Autodesk Inventor part; units mm, degrees
ref_plane "Start plane" through (0, 0, 0) normal (0, 0, 1) x (1, 0, 0)
ref_plane "End plane" through (0, 0, 300) normal (0, 0, 1) x (1, 0, 0)
ref_plane "Work Plane4" through (10, 0, 0) normal (-0.7071, 0, -0.7071) x (-0.7071, 0, 0.7071)
ref_plane "Start plane" through (0, 0, 0) normal (0, 0, 1) x (1, 0, 0)
ref_plane "End plane" through (0, 0, 300) normal (0, 0, 1) x (1, 0, 0)
sketch "Sketch" plane through (0, 0, 0) normal (0, 0, 1) x (1, 0, 0)
  line L0 (-10, -6) -> (-10, 6)
  line L1 (-6, 10) -> (6, 10)
  line L2 (10, 6) -> (10, -6)
  line L3 (6, -10) -> (-6, -10)
  arc A0 (-10, -6) -> (-6, -10) centre (-6, -6) ccw
  arc A1 (10, 6) -> (6, 10) centre (6, 6) ccw
  arc A2 (-6, 10) -> (-10, 6) centre (-6, 6) ccw
  arc A3 (6, -10) -> (10, -6) centre (6, -6) ccw
  arc A4 (-6, 8) -> (-8, 6) centre (-6, 6) ccw
  line L4 (-6, 8) -> (6, 8)
  arc A5 (8, 6) -> (6, 8) centre (6, 6) ccw
  line L5 (8, 6) -> (8, -6)
  arc A6 (6, -8) -> (8, -6) centre (6, -6) ccw
  line L6 (6, -8) -> (-6, -8)
  arc A7 (-8, -6) -> (-6, -8) centre (-6, -6) ccw
  line L7 (-8, -6) -> (-8, 6)
  line L8 (0, 15.1598) -> (0, -15.1598) construction
  line L9 (-15.1598, 0) -> (15.1598, 0) construction
  dimension "d7" = 4
  dimension "d9" = 20
  dimension "d11" = 20
  dimension "d12" = 2
  dimension "d15" = 10
  dimension "d16" = 10
extrude "Body" add sketch "Sketch" along normal up to surface (300 mm away) from surface at 0
sketch "Sketch3" plane through (0, 0, 0) normal (0, 0, 1) x (1, 0, 0)
  line L0 (0, 0) -> (10, 0)
ref_plane "Work Plane3" through (0, 0, 0) normal (0, -1, 0) x (1, 0, 0)
sketch "Sketch4" plane through (0, 0, 0) normal (0, -1, 0) x (1, 0, 0)
  line L0 (-2, 0) -> (12, 0)
  line L1 (-2, 300) -> (12, 300)
  dimension "d18" = 300
ref_plane "Work Plane4" through (10, 0, 0) normal (-0.7071, 0, -0.7071) x (-0.7071, 0, 0.7071)
split "Split1" plane through (10, 0, 0) removes the side toward (-0.7071, 0, -0.7071)
ref_plane "Work Plane5" through (10, 0, 300) normal (-0.7071, 0, 0.7071) x (0.7071, 0, 0.7071)
split "Split2" plane through (10, 0, 300) removes the side toward (-0.7071, 0, 0.7071)
equation "\"d7\" = G_IR"
equation "\"d9\" = G_W"
equation "\"d11\" = G_H"
equation "\"d12\" = G_T"
equation "\"d15\" = 0.5 * d9"
equation "\"d16\" = 0.5 * d11"
equation "\"d3\" = G_L"
equation "\"G_W\" = 20"
equation "\"G_H\" = 20"
equation "\"G_T\" = 2"
equation "\"G_IR\" = 4"
equation "\"G_L\" = d18"
equation "\"G_OFFSET_START\" = 0"
equation "\"G_OFFSET_END\" = 0"
properties part number "ISO 4019 - 20x20x2 - 300" material "Steel, Mild"
Geometry: final body of the model. Coordinates: model frame, mm. A direction names the side the tool comes from. Coordinates: 2 decimals unless noted, no trailing zeros. Loops run counter-clockwise (first coordinate to the right, second up) from the corner with the lowest first, then second, coordinate; pieces in that order, holes last. Notation, with made-up numbers: (-37, 86.25) - (-2, 86.25) arc R29 ccw to (-2, 113.25) - close; hole circle Ø9 at (84.5, -2.5). An arc over 180 degrees is marked (long way). One line per question, with ' | ' between items. Start each with the question number.
(1) Ray query, L1, parallel to Y at x = -0.5, z = 131; L2, parallel to Y at x = -7.5, z = 79. Return the intervals inside material, ascending. Write a range as from..to.
(2) Draft query along X for faces 1 (the flat face through (0, -10, 148)), 2 (the flat face through (-10, 0, 148)), 3 (the flat face through (0, -8, 148)). Return one class per face: +X half, -X half, draft (parallel to the pull), parting line (faces both ways), or undercut.
(3) First-contact query: pin 1 (2 mm diameter, centred on x = 2, y = -6.5, fed in from -Z); pin 2 (6 mm diameter, centred on x = 6, y = 2.5, fed in from +Z); pin 3 (2 mm diameter, centred on x = -6.5, z = 71.5, fed in from -Y). Flat tips, straight axial feed; report the tip coordinate or a pass-through.
(4) Cut plane C-C on z = 243. Output: boundary loops of the cut face in (x, y).
(5) Reachability of faces 4 (the flat face through (8, 0, 148)), 5 (the flat face through (0, 8.2, 10)) from +Z, -Z, +X, -X, +Y, -Y: full face, straight path, thin tool, end or side. Return the list, or none.
(6) Cut plane A-A on x = 3. Output: boundary loops of the cut face in (y, z).
(7) Cut plane B-B on y = 0.75. Output: boundary loops of the cut face in (x, z), and give its area (3 significant figures).
Here are the results:
1) L1: -10..-8, 8..10 | L2: -9.71..-7.32, 7.32..9.71
2) face 1: draft | face 2: -X half | face 3: undercut
3) pin 1: through | pin 2: z = 299 | pin 3: y = -10
4) outline: (-10, -6) arc R4 ccw to (-6, -10) - (6, -10) arc R4 ccw to (10, -6) - (10, 6) arc R4 ccw to (6, 10) - (-6, 10) arc R4 ccw to (-10, 6) - close; hole (-8, -6) arc R2 ccw to (-6, -8) - (6, -8) arc R2 ccw to (8, -6) - (8, 6) arc R2 ccw to (6, 8) - (-6, 8) arc R2 ccw to (-8, 6) - close
5) face 4: +Z, -Z | face 5: -Z, -X, +Y, -Y
6) outline: (-10, 7) - (-8, 7) - (-8, 293) - (-10, 293) - close; (8, 7) - (10, 7) - (10, 293) - (8, 293) - close
7) outline: (-10, 20) - (-8, 18) - (-8, 282) - (-10, 280) - close; (8, 2) - (10, 0) - (10, 300) - (8, 298) - close | area: 1,120 mm²
